Verification items for the finished model (mm, model axes). Give positions to 0.01 mm unless a question says otherwise; leave off trailing zeros. Write each loop counter-clockwise with the first axis right and the second up, starting at its lowest first coordinate (ties: lowest second). Pieces come first, ordered by that corner, then holes. Notation, with made-up numbers: M 66,68.25 L 106,68.25 A24 ccw 106,102.25 Z; hole C 10.25,66.25 d5. An arc over 180 degrees is marked long. Answer as a JSON object with one key per item and string values.
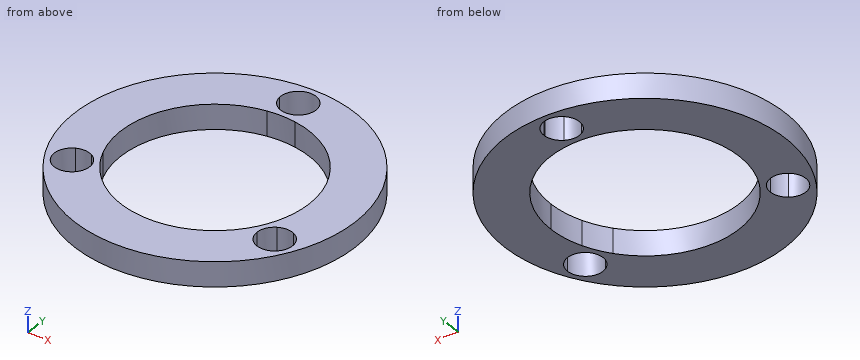
```python
from build123d import *

# Parameters (mm, degrees)
F0_R     = 45.5
F1_DEPTH = 8


with BuildPart() as f1:
    # F0 (on Top) → F1 (new body)
    with BuildSketch(Plane.XY):
        Circle(F0_R)
        with BuildLine():
            ThreePointArc((5.7335195457, 37.5649671053), (28.825975636, 24.7601116442), (38, 0))
            ThreePointArc((38, 0), (37.3440830117, -7.0298978664), (35.3989755783, -13.817109973))
            ThreePointArc((35.3989755783, -13.817109973), (37.7762057759, -15.9385509026), (38.6589653438, -19))
            ThreePointArc((38.6589653438, -19), (35.5933946557, -24.0849129068), (29.6654560327, -23.7478571323))
            ThreePointArc((29.6654560327, -23.7478571323), (0, -38), (-29.6654560327, -23.7478571323))
            ThreePointArc((-29.6654560327, -23.7478571323), (-37.8886114156, -21.875), (-35.3989755783, -13.817109973))
            ThreePointArc((-35.3989755783, -13.817109973), (-32.9089653438, 19), (-5.7335195457, 37.5649671053))
            ThreePointArc((-5.7335195457, 37.5649671053), (-0.2176724746, 43.7458784092), (5.75, 38))
            ThreePointArc((5.75, 38), (5.7458784092, 37.7823275254), (5.7335195457, 37.5649671053))
        make_face(mode=Mode.SUBTRACT)
        with BuildLine():
            ThreePointArc((35.3989755783, -13.817109973), (37.3440830117, -7.0298978664), (38, 0))
            ThreePointArc((38, 0), (28.825975636, 24.7601116442), (5.7335195457, 37.5649671053))
            ThreePointArc((5.7335195457, 37.5649671053), (4.8672404321, 34.9385509026), (2.875, 33.0203539282))
            Line((2.875, 33.0203539282), (4.5250023815, 30.1624659709))
            ThreePointArc((4.5250023815, 30.1624659709), (23.1112804993, 19.9027313121), (30.5, 0))
            ThreePointArc((30.5, 0), (29.9663216824, -5.6806306713), (28.3839629623, -11.1624659709))
            Line((28.3839629623, -11.1624659709), (30.0339653438, -14.0203539282))
            ThreePointArc((30.0339653438, -14.0203539282), (32.6912928692, -13.2541215908), (35.3989755783, -13.817109973))
        make_face()
        with BuildLine():
            ThreePointArc((-2.875, 33.0203539282), (-4.8672404321, 34.9385509026), (-5.7335195457, 37.5649671053))
            ThreePointArc((-5.7335195457, 37.5649671053), (-32.9089653438, 19), (-35.3989755783, -13.817109973))
            ThreePointArc((-35.3989755783, -13.817109973), (-32.6912928692, -13.2541215908), (-30.0339653438, -14.0203539282))
            Line((-30.0339653438, -14.0203539282), (-28.3839629623, -11.1624659709))
            ThreePointArc((-28.3839629623, -11.1624659709), (-26.4137748154, 15.25), (-4.5250023815, 30.1624659709))
            Line((-4.5250023815, 30.1624659709), (-2.875, 33.0203539282))
        make_face()
        with BuildLine():
            ThreePointArc((-29.6654560327, -23.7478571323), (0, -38), (29.6654560327, -23.7478571323))
            ThreePointArc((29.6654560327, -23.7478571323), (27.824052437, -21.6844293119), (27.1589653438, -19))
            Line((27.1589653438, -19), (23.8589605809, -19))
            ThreePointArc((23.8589605809, -19), (0, -30.5), (-23.8589605809, -19))
            Line((-23.8589605809, -19), (-27.1589653438, -19))
            ThreePointArc((-27.1589653438, -19), (-27.824052437, -21.6844293119), (-29.6654560327, -23.7478571323))
        make_face()
        with BuildLine():
            Line((4.5250023815, 30.1624659709), (2.875, 33.0203539282))
            ThreePointArc((2.875, 33.0203539282), (0, 32.25), (-2.875, 33.0203539282))
            Line((-2.875, 33.0203539282), (-4.5250023815, 30.1624659709))
            ThreePointArc((-4.5250023815, 30.1624659709), (0, 30.5), (4.5250023815, 30.1624659709))
        make_face()
        with BuildLine():
            ThreePointArc((27.1589653438, -19), (27.929319272, -16.125), (30.0339653438, -14.0203539282))
            Line((30.0339653438, -14.0203539282), (28.3839629623, -11.1624659709))
            ThreePointArc((28.3839629623, -11.1624659709), (26.4137748154, -15.25), (23.8589605809, -19))
            Line((23.8589605809, -19), (27.1589653438, -19))
        make_face()
        with BuildLine():
            Line((-28.3839629623, -11.1624659709), (-30.0339653438, -14.0203539282))
            ThreePointArc((-30.0339653438, -14.0203539282), (-27.929319272, -16.125), (-27.1589653438, -19))
            Line((-27.1589653438, -19), (-23.8589605809, -19))
            ThreePointArc((-23.8589605809, -19), (-26.4137748154, -15.25), (-28.3839629623, -11.1624659709))
        make_face()
    extrude(amount=F1_DEPTH)


solid = f1.part
```
1) Section check A-A on x = 0. Record the boundary of the cut face in (y, z).
Completed:
{"outline": "M -45.5,0 L -30.5,0 L -30.5,8 L -45.5,8 Z; M 30.5,0 L 32.25,0 L 32.25,8 L 30.5,8 Z; M 43.75,0 L 45.5,0 L 45.5,8 L 43.75,8 Z"}
2) Go/stop test with flat-tipped pins: pin 1 (8 mm diameter, centred on x = 6.5, y = -26.5, fed in from +Z); pin 2 (1 mm diameter, centred on y = 28, z = 4, fed in from -X); pin 3 (2 mm diameter, centred on y = 32, z = 5, fed in from -X); pin 4 (1 mm diameter, centred on x = -23.5, z = 2, fed in from +Y). Record where each tip stops, or that it passes through.
Completed:
{"pin 1": "stops at z = 8", "pin 2": "stops at x = -36.25", "pin 3": "stops at x = -33.31", "pin 4": "stops at y = 39.26"}
3) Section check B-B on y = 25. Record the boundary of the cut face in (x, z), and give its area (3 significant figures).
Completed:
{"outline": "M -38.02,0 L -17.47,0 L -17.47,8 L -38.02,8 Z; M 17.47,0 L 38.02,0 L 38.02,8 L 17.47,8 Z", "area": "329 mm2"}
4) Section check D-D on z = 1.75. Record the boundary of the cut face in (x, y) (3 decimals).
Completed:
{"outline": "C 0,0 d91; hole C -32.909,-19 d11.5; hole C 0,0 d61; hole C 0,38 d11.5; hole C 32.909,-19 d11.5"}
5) Section check C-C on x = -19.5. Record the boundary of the cut face in (y, z), and give its area (3 significant figures).
Completed:
{"outline": "M -41.11,0 L -23.45,0 L -23.45,8 L -41.11,8 Z; M 23.45,0 L 41.11,0 L 41.11,8 L 23.45,8 Z", "area": "283 mm2"}
6) Thickness scan on L1, parallel to X at y = -21, z = 2.75; L2, parallel to X at y = 15, z = 5.25; L3, parallel to Y at x = 1, z = 6.75. Record the ranges inside material, lowest first.
Completed:
{"L1": "x = -40.36 to -38.3, -27.52 to -22.12, 22.12 to 27.52, 38.3 to 40.36", "L2": "x = -42.96 to -26.56, 26.56 to 42.96", "L3": "y = -45.49 to -30.48, 30.48 to 32.34, 43.66 to 45.49"}
